```python
from build123d import *

# Parameters (mm, degrees)
F0_W      = 25.4
F0_H      = 18.542
F1_DEPTH  = 1.8034
F2_R      = 4.572
F3_DEPTH  = 3.3655
F3_FACE_R = 4.572
F4_DEPTH  = 1.5621


with BuildPart() as f1:
    # F0 (on Top) → F1 (new body)
    with BuildSketch(Plane.XY):
        with Locations((-41.440347, 17.31006)):
            Rectangle(F0_W, F0_H)
    extrude(amount=F1_DEPTH)

    # F2 (on face) → F3 (join, symmetric)
    with BuildSketch(Plane.XY.offset(1.8034)):
        with Locations((-41.445623, 17.31006)):
            Circle(F2_R)
    extrude(amount=F3_DEPTH, both=True)

    # F3_face (on face) → F4 (cut, through all)
    with BuildSketch(Plane(origin=(-41.445623, 17.31006, -1.5621), x_dir=(1, 0, 0), z_dir=(0, 0, -1))):
        Circle(F3_FACE_R)
    extrude(amount=-F4_DEPTH, mode=Mode.SUBTRACT)


solid = f1.part
```
Input: part model. Units: mm. Frame: model coordinates. A direction names the side the tool comes from. Round coordinates to 2 decimals unless told otherwise and drop trailing zeros. Write each loop counter-clockwise with the first axis right and the second up, starting at its lowest first coordinate (ties: lowest second). Pieces come first, ordered by that corner, then holes. Notation, with made-up numbers: (-4, 26.5) -> (39, 26.5) arc R33 ccw to (39, 65.5) -> close; hole circle Ø8 at (-14, 52). An arc over 180 degrees is marked (long way). Answer as CSV lines item,"result".
1. Section C-C (x = -49.25). Return the cut outline in (y, z).
Geometry says:
outline,"(8.04, 0) -> (26.58, 0) -> (26.58, 1.8) -> (8.04, 1.8) -> close"
2. Contact query for a flat-ended pin moving along its axis: P1, Ø3, axis at y = 24.5, z = 4, coming from the +X side. Output: stop coordinate, or through.
Geometry says:
P1,"passes through"
3. Reachability of faces 1 (the cylindrical face through (-37.085, 18.683, 3.51)), 2 (the flat face through (-42, 17, 0)) from +Z, -Z, +X, -X, +Y, -Y: full face, straight path, thin tool, end or side. Return the list, or none.
Geometry says:
face 1,"+Z"
face 2,"-Z, +X, -X, +Y, -Y"
4. Section D-D (z = 3.7). Return the cut outline in (x, y), plus the area to 3 significant figures.
Geometry says:
outline,"circle Ø9.14 at (-41.45, 17.31)"
area,"65.7 mm^2"
5. Section B-B (x = -42). Return the cut outline in (y, z).
Geometry says:
outline,"(8.04, 0) -> (26.58, 0) -> (26.58, 1.8) -> (21.85, 1.8) -> (21.85, 5.17) -> (12.77, 5.17) -> (12.77, 1.8) -> (8.04, 1.8) -> close"
6. Section A-A (y = 21.5). Return the cut outline in (x, z), plus the area to 3 significant figures.
Geometry says:
outline,"(-54.14, 0) -> (-28.74, 0) -> (-28.74, 1.8) -> (-39.62, 1.8) -> (-39.62, 5.17) -> (-43.28, 5.17) -> (-43.28, 1.8) -> (-54.14, 1.8) -> close"
area,"58.1 mm^2"
7. Ray query, L1, parallel to Z at x = -38.75, y = 11.25; L2, parallel to X at y = 21, z = 3.95; L3, parallel to X at y = 18.5, z = 3.15. Return the intervals inside material, ascending. Write a range as [from, to].
Geometry says:
L1,"z = [0, 1.8]"
L2,"x = [-44.15, -38.75]"
L3,"x = [-45.86, -37.03]"
